For this review, take the finished solid that the model builds, in its own axes (mm). Round coordinates to 2 decimals unless told otherwise and drop trailing zeros. Order: outer loops, then holes, each group sorted by start corner. A loop starts at its lowest first (then second) coordinate and runs counter-clockwise, first axis right, second up. Notation, with made-up numbers: M 10.25,-13 L 24.25,-13 A22 ccw 24.25,-6 Z; hole C 45.5,74.5 d1. An arc over 180 degrees is marked long. Use a Markdown table: item, result.
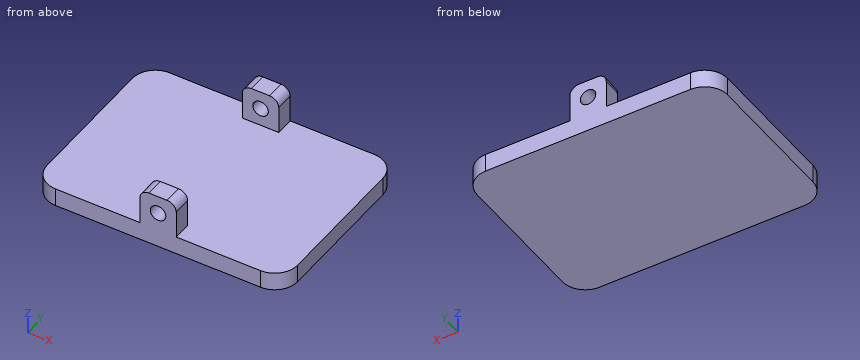
from build123d import *

# Parameters (mm, degrees)
MIRROREDSKETCH_W = 8
MIRROREDSKETCH_H = 4
PAD002_DEPTH     = 8
SKETCH_W         = 55
SKETCH_H         = 40
PAD_DEPTH        = 4
SKETCH001_W      = 8
SKETCH001_H      = 4
PAD001_DEPTH     = 8
SKETCH002_R      = 1.7
POCKET_DEPTH     = 40.001
FILLET_R         = 2
FILLET001_R      = 5


with BuildPart() as pad002:
    # MirroredSketch → Pad002 (new body)
    with BuildSketch(Plane.XY.offset(4)):
        with Locations((0, -18)):
            Rectangle(MIRROREDSKETCH_W, MIRROREDSKETCH_H)
    extrude(amount=PAD002_DEPTH)


with BuildPart() as fillet001:
    # Sketch → Pad (new body)
    with BuildSketch(Plane.XY):
        Rectangle(SKETCH_W, SKETCH_H)
    extrude(amount=PAD_DEPTH)

    # Sketch001 → Pad001 (new body)
    with BuildSketch(Plane.XY.offset(4)):
        with Locations((0, 18)):
            Rectangle(SKETCH001_W, SKETCH001_H)
    extrude(amount=PAD001_DEPTH)

    # Fusion: union Pad002
    add(pad002.part)

    # Sketch002 → Pocket (cut, through all)
    with BuildSketch(Plane.XZ.offset(20)):
        with Locations((0, 8)):
            Circle(SKETCH002_R)
    extrude(amount=-POCKET_DEPTH, mode=Mode.SUBTRACT)

    # Fillet
    fillet_edges = [fillet001.edges().sort_by_distance(p)[0] for p in [
        (4, -18, 12),
        (-4, -18, 12),
        (4, 18, 12),
        (-4, 18, 12),
    ]]
    fillet(fillet_edges, radius=FILLET_R)

    # Fillet001
    fillet001_edges = [fillet001.edges().sort_by_distance(p)[0] for p in [
        (27.5, 20, 2),
        (-27.5, 20, 2),
        (27.5, -20, 2),
        (-27.5, -20, 2),
    ]]
    fillet(fillet001_edges, radius=FILLET001_R)


solid = fillet001.part
Q1. Add section C-C (z = 4.75). Write out the cut boundary in (x, y).
Determined:
| item | result |
|---|---|
| outline | M -4,-20 L 4,-20 L 4,-16 L -4,-16 Z; M -4,16 L 4,16 L 4,20 L -4,20 Z |
Q2. Wall thickness on line 1 along Z through (x, y) = (0, 18.1); line 2 along Z through (x, y) = (19.5, 8.5); line 3 along Y through (x, z) = (-1.5, 4.25): over which ranges is each line inside the solid? List them lowest first. Write a range as [from, to].
Determined:
| item | result |
|---|---|
| line 1 | z = [0, 6.3], [9.7, 12] |
| line 2 | z = [0, 4] |
| line 3 | y = [-20, -16], [16, 20] |
Q3. Clearance check with flat-ended pins moving along their axes: pin 1 (2 mm diameter, centred on y = -17.5, z = 8, fed in from +X); pin 2 (6 mm diameter, centred on y = 5.5, z = 9, fed in from -X); pin 3 (1.2 mm diameter, centred on y = 17.5, z = 6.5, fed in from -X). State where each tip first meets the part, or that it passes through.
Determined:
| item | result |
|---|---|
| pin 1 | stops at x = 4 |
| pin 2 | passes through |
| pin 3 | stops at x = -4 |
Q4. Add section B-B (x = 0). Write out the cut boundary in (y, z), then the cut area to 3 significant figures.
Determined:
| item | result |
|---|---|
| outline | M -20,0 L 20,0 L 20,6.3 L 16,6.3 L 16,4 L -16,4 L -16,6.3 L -20,6.3 Z; M -20,9.7 L -16,9.7 L -16,12 L -20,12 Z; M 16,9.7 L 20,9.7 L 20,12 L 16,12 Z |
| area | 197 mm^2 |
Q5. Add section A-A (z = 8). Write out the cut boundary in (x, y), then the cut area to 3 significant figures.
Determined:
| item | result |
|---|---|
| outline | M -4,-20 L -1.7,-20 L -1.7,-16 L -4,-16 Z; M -4,16 L -1.7,16 L -1.7,20 L -4,20 Z; M 1.7,-20 L 4,-20 L 4,-16 L 1.7,-16 Z; M 1.7,16 L 4,16 L 4,20 L 1.7,20 Z |
| area | 36.8 mm^2 |
Q6. Add section D-D (z = 11). Write out the cut boundary in (x, y).
Determined:
| item | result |
|---|---|
| outline | M -3.73,-20 L 3.73,-20 L 3.73,-16 L -3.73,-16 Z; M -3.73,16 L 3.73,16 L 3.73,20 L -3.73,20 Z |
